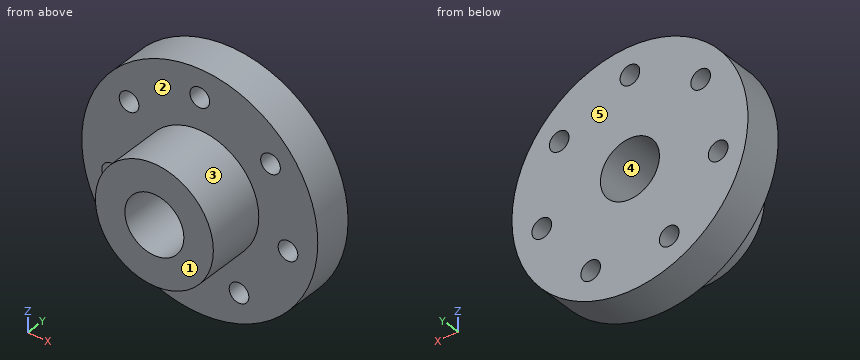
from build123d import *

# Parameters (mm, degrees)
F0_R            = 38.1
F0_R_2          = 19.05
F1_DEPTH        = 12.7
F0_R_3          = 9.525
F2_DEPTH        = 31.75
F3_R            = 3.175
F4_DEPTH        = 12.701
F4_COPIES_COUNT = 7


# Not quite as in the source:
# - a pattern or mirror of a feature is missing from the dataset's text; its kind, count and spacing are read off the source's solid


with BuildPart() as f1:
    # F0 (on Front) → F1 (new body)
    with BuildSketch(Plane.XZ):
        Circle(F0_R)
        Circle(F0_R_2, mode=Mode.SUBTRACT)
    extrude(amount=F1_DEPTH)

    # F0 (on Front) → F2 (join)
    with BuildSketch(Plane.XZ):
        Circle(F0_R_2)
        Circle(F0_R_3, mode=Mode.SUBTRACT)
    extrude(amount=F2_DEPTH)

    # F3 (on face) → F4 (cut, through all)
    with BuildSketch(Plane.XZ.offset(12.7)):
        with Locations((0, 29.21)):
            Circle(F3_R)
    f4 = extrude(amount=-F4_DEPTH, mode=Mode.SUBTRACT)

    # F4_copies: F4 ×7 about axis
    f4_copies_axis = Axis((0, 0, 0), (0, 1, 0))
    for i in range(1, F4_COPIES_COUNT):
        add(f4.rotate(f4_copies_axis, i * 360 / F4_COPIES_COUNT), mode=Mode.SUBTRACT)


solid = f1.part
The model under review builds one solid part; all positions refer to its coordinate system, in mm. Face numbers are marked on the shaded views. A direction names the side the tool comes from. Round coordinates to 2 decimals unless told otherwise and drop trailing zeros. Order: outer loops, then holes, each group sorted by start corner. A loop starts at its lowest first (then second) coordinate and runs counter-clockwise, first axis right, second up. Notation, with made-up numbers: (38.25, 68) -> (60.25, 68) arc R14 cw to (60.25, 75) -> close; hole circle Ø3 at (89.25, 35.5). An arc over 180 degrees is marked (long way). Return JSON: item names as keys, results as strings.
1. For L1, parallel to Y at x = -25.5, z = 5.5; L2, parallel to Z at x = 14, y = -9.5; L3, parallel to Z at x = 2, y = -2.5, list the stretches that pass through material, from the lowest coordinate up. Write a range as [from, to].
Answer block:
{"L1": "y = [-12.7, 0]", "L2": "z = [-35.43, -29.2], [-23.43, 35.43]", "L3": "z = [-38.05, -9.31], [9.31, 26.74], [31.68, 38.05]"}
2. Take a section at D-D (x = 13.5). Write out the cut boundary in (y, z), then the cut area to 3 significant figures.
Answer block:
{"outline": "(-31.75, -13.44) -> (-12.7, -13.44) -> (-12.7, -23.25) -> (0, -23.25) -> (0, 35.63) -> (-12.7, 35.63) -> (-12.7, 13.44) -> (-31.75, 13.44) -> close; (-12.7, -35.63) -> (0, -35.63) -> (0, -29.38) -> (-12.7, -29.38) -> close", "area": "1,340 mm²"}
3. Take a section at B-B (x = 0). Write out the cut boundary in (y, z) (3 decimals).
Answer block:
{"outline": "(-31.75, -19.05) -> (-12.7, -19.05) -> (-12.7, -38.1) -> (0, -38.1) -> (0, -9.525) -> (-31.75, -9.525) -> close; (-31.75, 9.525) -> (0, 9.525) -> (0, 26.035) -> (-12.7, 26.035) -> (-12.7, 19.05) -> (-31.75, 19.05) -> close; (-12.7, 32.385) -> (0, 32.385) -> (0, 38.1) -> (-12.7, 38.1) -> close"}
4. The part is to be moulded in two halves that separate along Z. For the marked faces 3, 4 and 5, say which applies: +Z half, -Z half, draft (parallel to the pull), parting line (faces both ways), or undercut.
Answer block:
{"face 3": "parting line", "face 4": "undercut", "face 5": "draft"}
5. For the marked faces 1 and 2, list the 3-axis set-ups (+Z, -Z, +X, -X, +Y, -Y) from which the entire face can be reached by the end or side of a thin tool; tool diameter is ignored.
Answer block:
{"face 1": "+Z, -Z, +X, -X, -Y", "face 2": "-Y"}
6. Take a section at A-A (z = 0). Write out the cut boundary in (x, y) (3 decimals).
Answer block:
{"outline": "(-38.1, -12.7) -> (-19.05, -12.7) -> (-19.05, -31.75) -> (-9.525, -31.75) -> (-9.525, 0) -> (-38.1, 0) -> close; (9.525, -31.75) -> (19.05, -31.75) -> (19.05, -12.7) -> (38.1, -12.7) -> (38.1, 0) -> (9.525, 0) -> close"}
7. Take a section at C-C (y = -2.5). State how many separate pieces and enclosed holes the cut face has, then the cut area to 3 significant figures.
Answer block:
{"separate pieces": "1", "enclosed holes": "8", "area": "4,050 mm²"}
8. Insertion check: P1, Ø12, axis at y = -8.5, z = 26, coming from the +X side; P2, Ø7.5, axis at x = 22.84, z = 18.21, coming from the -Y side; P3, Ø10, axis at x = 0, z = 29.21, coming from the +Y side; P4, Ø6, axis at x = 15, y = -14, coming from the -Z side. Each pin has a flat end and moves straight along its axis. Give the tip position at first contact, or say it passes through.
Answer block:
{"P1": "stops at x = 32.43", "P2": "stops at y = -12.7", "P3": "stops at y = 0", "P4": "stops at z = -36.06"}
